```python
from build123d import *

# Parameters (mm, degrees)
SKETCH_1_W          = 27
SKETCH_1_H          = 5
EXTRUDE_1_DEPTH     = 8
SKETCH_2_W          = 3
SKETCH_2_H          = 5
EXTRUDE_2_DEPTH     = 13
SKETCH_3_R          = 0.5
CUT_EXTRUDE_1_DEPTH = 3
SKETCH_4_R          = 1.5
SKETCH_4_R_2        = 1
EXTRUDE_3_DEPTH     = 4
SKETCH_6_R          = 2
EXTRUDE_5_DEPTH     = 2
SKETCH_7_W          = 7.5
SKETCH_7_H          = 1.5
EXTRUDE_6_DEPTH     = 10
FILLET_1_R          = 1.5


with BuildPart() as part:
    # 草图1 → 凸台-拉伸1 (new body)
    with BuildSketch(Plane.XY):
        Rectangle(SKETCH_1_W, SKETCH_1_H)
    extrude(amount=EXTRUDE_1_DEPTH)

    # 草图2 → 凸台-拉伸2 (add)
    with BuildSketch(Plane(origin=(0, 0, 0), x_dir=(-1, 0, 0), z_dir=(0, 0, -1))):
        with Locations((-12, 0)):
            Rectangle(SKETCH_2_W, SKETCH_2_H)
    extrude(amount=EXTRUDE_2_DEPTH)

    # 草图3 → 切除-拉伸1 (cut)
    with BuildSketch(Plane(origin=(0, 0, -13), x_dir=(-1, 0, 0), z_dir=(0, 0, -1))):
        with Locations((-12, 1.3)):
            Circle(SKETCH_3_R)
        with Locations(Location((-12, -1.3, 0), (0, 0, 180))):
            Circle(SKETCH_3_R)
    extrude(amount=-CUT_EXTRUDE_1_DEPTH, mode=Mode.SUBTRACT)

    # 草图4 → 凸台-拉伸3 (add)
    with BuildSketch(Plane(origin=(13.5, 0, 0), x_dir=(0, 0, -1), z_dir=(1, 0, 0))):
        with Locations(Location((-6, 0, 0), (0, 0, 180))):
            Circle(SKETCH_4_R)
        with Locations((-6, 0)):
            Circle(SKETCH_4_R_2, mode=Mode.SUBTRACT)
    extrude(amount=EXTRUDE_3_DEPTH)

    # 草图6 → 凸台-拉伸5 (add)
    with BuildSketch(Plane.ZY.offset(-1)):
        with BuildLine():
            Line((8, 2.5), (0, 2.5))
            Line((0, 2.5), (0, 5.5))
            ThreePointArc((0, 5.5), (4, 9.5), (8, 5.5))
            Line((8, 5.5), (8, 2.5))
        make_face()
        with Locations((4, 5.5)):
            Circle(SKETCH_6_R, mode=Mode.SUBTRACT)
    extrude(amount=-EXTRUDE_5_DEPTH)

    # 草图7 → 凸台-拉伸6 (add)
    with BuildSketch(Plane(origin=(0, 0, 0), x_dir=(-1, 0, 0), z_dir=(0, 0, -1))):
        with Locations((-3.5, 0)):
            Rectangle(SKETCH_7_W, SKETCH_7_H)
        with Locations((8, 0)):
            Rectangle(SKETCH_7_W, SKETCH_7_H)
    extrude(amount=EXTRUDE_6_DEPTH)

    # 圆角1
    fillet_1_edges = [part.edges().sort_by_distance(p)[0] for p in [
        (7.25, 0, -10),
        (-0.25, 0, -10),
        (-4.25, 0, -10),
        (-11.75, 0, -10),
    ]]
    fillet(fillet_1_edges, radius=FILLET_1_R)


solid = part.part
```
The listing builds one solid part. Answer for the finished solid, in the listing's coordinates (mm). A direction names the side the tool comes from. Give positions to 0.01 mm unless a question says otherwise; leave off trailing zeros. Write each loop counter-clockwise with the first axis right and the second up, starting at its lowest first coordinate (ties: lowest second). Pieces come first, ordered by that corner, then holes. Notation, with made-up numbers: (28.25, -2) -> (37.25, -2) arc R15 ccw to (37.25, 27) -> close; hole circle Ø8 at (85, -34.5). An arc over 180 degrees is marked (long way). Use one line per item in the form item = value.
1) Each of these flat-tipped pins is pushed along its axis until it touches: P1, Ø6, axis at x = -6.5, z = -5, coming from the +Y side; P2, Ø12, axis at x = 11.5, z = -3, coming from the +Y side; P3, Ø5, axis at y = 4.5, z = -2, coming from the +X side. Where does it stop, or does it pass through?
Result:
P1 = 0.75
P2 = 2.5
P3 = 13.5
2) A tool of negligible diameter and unlimited length cuts with its end or side. For faces 4 (the flat face through (1, 8, 4)), 5 (the cylindrical face through (15.47, -0.07, 4.5)), 6 (the flat face through (-8, 0.75, -5)), from which of +Z, -Z, +X, -X, +Y, -Y can it reach the whole face along a straight path? Write none if from no direction.
Result:
face_4 = +Z, -Z, -X, +Y
face_5 = +X
face_6 = -Z, -X, +Y
3) Straight lines are drawn through the part: probe 1 along Y at (x, z) = (12, -11.05); probe 2 along Y at (x, z) = (1.65, 4); probe 3 along Z at (x, y) = (-5.5, 1.25). For each, find the intervals that lie inside material, in ascending order.
Result:
probe_1 = -2.5 to -1.8, -0.8 to 0.8, 1.8 to 2.5
probe_2 = -2.5 to 3.5, 7.5 to 9.5
probe_3 = 0 to 8
4) Section D-D on x = 12 is taken. Write down the section's boundary in (y, z).
Result:
outline = (-2.5, -13) -> (-1.8, -13) -> (-1.8, -10) -> (-0.8, -10) -> (-0.8, -13) -> (0.8, -13) -> (0.8, -10) -> (1.8, -10) -> (1.8, -13) -> (2.5, -13) -> (2.5, 8) -> (-2.5, 8) -> close
5) For a pull along Y with two mould halves and no side action, classify faces 1 (the flat face through (10.5, 0, -6)), 2 (the flat face through (-6, 2.5, 4)), 3 (the flat face through (12, -1, -10)) as +Y half, -Y half, draft (parallel to the pull), parting line (faces both ways), or undercut.
Result:
face_1 = draft
face_2 = +Y half
face_3 = undercut
6) Section C-C on y = 4.25 is taken. Write down the section's boundary in (x, z).
Result:
outline = (1, 0) -> (3, 0) -> (3, 2.44) -> (1, 2.44) -> close; (1, 5.56) -> (3, 5.56) -> (3, 8) -> (1, 8) -> close
7) Section B-B on z = 4 is taken. Write down the section's boundary in (x, y), plus the area to 3 significant figures.
Result:
outline = (-13.5, -2.5) -> (13.5, -2.5) -> (13.5, 2.5) -> (3, 2.5) -> (3, 3.5) -> (1, 3.5) -> (1, 2.5) -> (-13.5, 2.5) -> close; (1, 7.5) -> (3, 7.5) -> (3, 9.5) -> (1, 9.5) -> close
area = 141 mm²
8) Section A-A on z = -2 is taken. Write down the section's boundary in (x, y).
Result:
outline = (-11.75, -0.75) -> (-4.25, -0.75) -> (-4.25, 0.75) -> (-11.75, 0.75) -> close; (-0.25, -0.75) -> (7.25, -0.75) -> (7.25, 0.75) -> (-0.25, 0.75) -> close; (10.5, -2.5) -> (13.5, -2.5) -> (13.5, 2.5) -> (10.5, 2.5) -> close
